Verification items for the finished model (mm, model axes). Face numbers are marked on the shaded views. A direction names the side the tool comes from. Give positions to 0.01 mm unless a question says otherwise; leave off trailing zeros. Loops run counter-clockwise (first coordinate to the right, second up) from the corner with the lowest first, then second, coordinate; pieces in that order, holes last. Notation, with made-up numbers: M -31,-10.5 L -14,-10.5 A25 cw -14,3.5 Z; hole C -0.5,67.5 d7. An arc over 180 degrees is marked long. Answer in a Markdown table with one row per item.
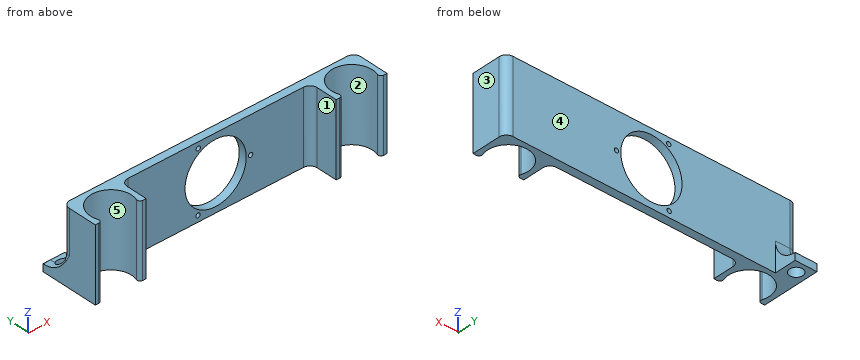
```python
from build123d import *

# Parameters (mm, degrees)
SKETCH1_R           = 14
BOSS_EXTRUDE1_DEPTH = 50
SKETCH2_R           = 21
CUT_EXTRUDE1_DEPTH  = 45
SKETCH3_R           = 1.5
CUT_EXTRUDE2_DEPTH  = 45
SKETCH4_W           = 15
SKETCH4_H           = 15
BOSS_EXTRUDE2_DEPTH = 5
SKETCH5_R           = 4.5
CUT_EXTRUDE3_DEPTH  = 5
FILLET1_R           = 5
FILLET2_R           = 15
SKETCH7_W           = 200
SKETCH7_H           = 10
CUT_EXTRUDE4_DEPTH  = 50
FILLET3_R           = 2


with BuildPart() as part:
    # Sketch1 → Boss-Extrude1 (new body)
    with BuildSketch(Plane.XY):
        Polygon((-50, 17.4), (-15.2, 17.4), (50, 17.4), (50, 12.022605171), (-15.17275181, 12.022605171), (-15.17275181, -17.4), (-50, -17.4), align=None)
        with Locations((-32.6, 0)):
            Circle(SKETCH1_R, mode=Mode.SUBTRACT)
    boss_extrude1 = extrude(amount=BOSS_EXTRUDE1_DEPTH)

    # Mirror1: Boss-Extrude1 across plane
    add(boss_extrude1.mirror(Plane(origin=(50, 17.4, 50), x_dir=(0, 0, 1), z_dir=(-1, 0, 0))))

    # Sketch2 → Cut-Extrude1 (cut)
    with BuildSketch(Plane(origin=(0, 17.4, 0), x_dir=(1, 0, 0), z_dir=(0, 1, 0))):
        with Locations(Location((50, -25, 0), (0, 0, 270))):
            Circle(SKETCH2_R)
    extrude(amount=-CUT_EXTRUDE1_DEPTH, mode=Mode.SUBTRACT)

    # Sketch3 → Cut-Extrude2 (cut)
    with BuildSketch(Plane(origin=(0, 17.4, 0), x_dir=(1, 0, 0), z_dir=(0, 1, 0))):
        with Locations(Location((37.89578471, -4.273302643, 0), (0, 0, 270))):
            Circle(SKETCH3_R)
        with Locations(Location((74.001954093, -24.880790745, 0), (0, 0, 270))):
            Circle(SKETCH3_R)
        with Locations(Location((38.102261197, -45.845906612, 0), (0, 0, 270))):
            Circle(SKETCH3_R)
    extrude(amount=-CUT_EXTRUDE2_DEPTH, mode=Mode.SUBTRACT)

    # Sketch4 → Boss-Extrude2 (add)
    with BuildSketch(Plane(origin=(0, 0, 0), x_dir=(-1, 0, 0), z_dir=(0, 0, -1))):
        with Locations((42.5, 24.9)):
            Rectangle(SKETCH4_W, SKETCH4_H)
    extrude(amount=-BOSS_EXTRUDE2_DEPTH)

    # Sketch5 → Cut-Extrude3 (cut)
    with BuildSketch(Plane(origin=(0, 0, 0), x_dir=(-1, 0, 0), z_dir=(0, 0, -1))):
        with Locations((42.5, 24.9)):
            Circle(SKETCH5_R)
    extrude(amount=-CUT_EXTRUDE3_DEPTH, mode=Mode.SUBTRACT)

    # Fillet1
    fillet1_edges = [part.edges().sort_by_distance(p)[0] for p in [
        (-50, 17.4, 27.5),
        (-15.17275181, 12.022605171, 25),
        (-15.17275181, -17.4, 25),
        (-50, -17.4, 25),
        (150, -17.4, 25),
        (150, 17.4, 25),
        (115.17275181, 12.022605171, 25),
        (115.17275181, -17.4, 25),
    ]]
    fillet(fillet1_edges, radius=FILLET1_R)

    # Fillet2
    # the kernel refuses this fillet: 15 mm, written as the material it adds along each edge
    with BuildSketch(Plane(origin=(-45, 12.4, 5), x_dir=(0, 1, 0), z_dir=(1, 0, 0))) as fillet2_piece_1_section:
        with BuildLine():
            CenterArc((5 + FILLET2_R, FILLET2_R), FILLET2_R, 180, 90)
            Line((5 + FILLET2_R, 0), (5, 0))
            Line((5, 0), (5, FILLET2_R))
        make_face()
    fillet2_piece_1 = revolve(axis=Axis((-45, 12.4, 5), (0, 0, 1)), revolution_arc=359.64, mode=Mode.PRIVATE)
    fillet2_piece_1 = split(fillet2_piece_1, bisect_by=Plane(origin=(-50, 16.22028394, 10.678167657), z_dir=(1, 0, 0)), keep=Keep.TOP, mode=Mode.PRIVATE)
    fillet2_piece_1 = fillet2_piece_1 - Plane(origin=(-42.5, 24.9, 10.678167657), x_dir=(-1, 0, 0), z_dir=(0, 0, -1)) * Cylinder(4.5, 80, mode=Mode.PRIVATE)
    fillet2_piece_1 = fillet2_piece_1 - Plane(origin=(-32.6, 0, 10.678167657), x_dir=(1, 0, 0), z_dir=(0, 0, -1)) * Cylinder(14, 80, mode=Mode.PRIVATE)
    fillet2_piece_1 = split(fillet2_piece_1, bisect_by=Plane(origin=(-35, 16.22028394, 10.678167657), z_dir=(-1, 0, 0)), keep=Keep.TOP, mode=Mode.PRIVATE)
    add(fillet2_piece_1)
    with BuildSketch(Plane(origin=(-45, 17.4, 5), x_dir=(0, 0, 1), z_dir=(1, 0, 0))) as fillet2_piece_2_section:
        with BuildLine():
            CenterArc((FILLET2_R, -FILLET2_R), FILLET2_R, 90, 90)
            Line((0, -FILLET2_R), (0, 0))
            Line((0, 0), (FILLET2_R, 0))
        make_face()
    fillet2_piece_2 = extrude(amount=10, mode=Mode.PRIVATE)
    fillet2_piece_2 = fillet2_piece_2 - Plane(origin=(-42.5, 24.9, 8.942844525), x_dir=(-1, 0, 0), z_dir=(0, 0, -1)) * Cylinder(4.5, 80, mode=Mode.PRIVATE)
    add(fillet2_piece_2)

    # Sketch7 → Cut-Extrude4 (cut)
    with BuildSketch(Plane(origin=(0, 0, 0), x_dir=(-1, 0, 0), z_dir=(0, 0, -1))):
        with Locations((-50, -12.4)):
            Rectangle(SKETCH7_W, SKETCH7_H)
    extrude(amount=-CUT_EXTRUDE4_DEPTH, mode=Mode.SUBTRACT)

    # Fillet3
    fillet3_edges = [part.edges().sort_by_distance(p)[0] for p in [
        (120.715556387, -7.4, 25),
        (144.484443613, -7.4, 25),
        (-20.715556387, -7.4, 25),
        (-44.484443613, -7.4, 25),
    ]]
    fillet(fillet3_edges, radius=FILLET3_R)


solid = part.part
```
Item 1: Sectioned sample at B-B (y = 1.5). Record the cut outline in (x, z).
Reported:
| item | result |
|---|---|
| outline | M -50,0 L -46.52,0 L -46.52,50 L -50,50 Z; M -18.68,0 L -15.17,0 L -15.17,50 L -18.68,50 Z; M 115.17,0 L 118.68,0 L 118.68,50 L 115.17,50 Z; M 146.52,0 L 150,0 L 150,50 L 146.52,50 Z |
Item 2: Go/stop test with flat-tipped pins: pin 1 (25 mm diameter, centred on x = 28, z = 30.5, fed in from -Y); pin 2 (3 mm diameter, centred on x = 96, z = 24, fed in from +Y); pin 3 (11.5 mm diameter, centred on x = -42.5, y = 24.9, fed in from +Z). Record where each tip stops, or that it passes through.
Reported:
| item | result |
|---|---|
| pin 1 | stops at y = 12.02 |
| pin 2 | stops at y = 17.4 |
| pin 3 | stops at z = 12.97 |
Item 3: Sectioned sample at D-D (x = 13.5). Record the cut outline in (y, z), and give its area (3 significant figures).
Reported:
| item | result |
|---|---|
| outline | M 12.02,0 L 17.4,0 L 17.4,50 L 12.02,50 Z |
| area | 269 mm^2 |
Item 4: Scan lines: L1, parallel to X at y = 0, z = 29.5; L2, parallel to X at y = 3.5, z = 21.5; L3, parallel to Y at x = 132.6, z = 21. Record each from-to range of solid material in increasing order. Write a range as [from, to].
Reported:
| item | result |
|---|---|
| L1 | x = [-50, -46.6], [-18.6, -15.17], [115.17, 118.6], [146.6, 150] |
| L2 | x = [-50, -46.16], [-19.04, -15.17], [115.17, 119.04], [146.16, 150] |
| L3 | y = [14, 17.4] |
Item 5: Sectioned sample at A-A (z = 8). Record the cut outline in (x, y) (3 decimals).
Reported:
| item | result |
|---|---|
| outline | M -50,-7.4 L -47.661,-7.4 A2 ccw -45.779,-4.725 A14 cw long -19.421,-4.725 A2 ccw -17.539,-7.4 L -15.173,-7.4 L -15.173,7.023 A5 cw -10.173,12.023 L 37.671,12.023 L 37.671,17.4 L -35,17.4 L -35,23.4 L -38.257,23.4 A4.5 cw -46.694,23.269 A11 ccw -50,22.198 Z; M 62.329,12.023 L 110.173,12.023 A5 cw 115.173,7.023 L 115.173,-7.4 L 117.539,-7.4 A2 ccw 119.421,-4.725 A14 cw long 145.779,-4.725 A2 ccw 147.661,-7.4 L 150,-7.4 L 150,12.4 A5 ccw 145,17.4 L 62.329,17.4 Z |
Item 6: Tool access check on the marked faces 1 and 2. Record the directions out of +Z, -Z, +X, -X, +Y, -Y that give a thin tool (end or side, any length) a straight path to the whole face; none if there is none.
Reported:
| item | result |
|---|---|
| face 1 | +Z, -Z, -Y |
| face 2 | +Z, -Z |
Item 7: Release check for a two-part mould opening along Y. For the marked faces 3, 4 and 5 record: released by +Y, released by -Y, zero draft, split by the parting line, or undercut.
Reported:
| item | result |
|---|---|
| face 3 | zero draft |
| face 4 | released by +Y |
| face 5 | undercut |
Item 8: Sectioned sample at C-C (x = -42.5). Record the cut outline in (y, z), and give its area (3 significant figures).
Reported:
| item | result |
|---|---|
| outline | M 9.9,0 L 20.4,0 L 20.4,11 A15 cw 17.4,20 L 17.4,50 L 9.9,50 Z; M 29.4,0 L 32.4,0 L 32.4,5 A15 cw 29.4,5.3 Z |
| area | 432 mm^2 |
